Study the drawing (mm; zero at the part's minimum x, y, z) and answer. A direction names the side the tool comes from. Round coordinates to 2 decimals unless told otherwise and drop trailing zeros. Loops run counter-clockwise (first coordinate to the right, second up) from the corner with the lowest first, then second, coordinate; pieces in that order, holes last. Notation, with made-up numbers: (-11, 7.25) - (4, 7.25) arc R30 ccw to (4, 31.25) - close; hole circle Ø7 at (2, 0.25). An arc over 180 degrees is marked (long way). Use CSV: the item, a comma, the result in double quotes. Start each with the question number.
1. Find section B-B (y = 56). Give the vertices of the cut face in (x, z).
2. Given pin 1 Ø10 at (y, z) = (83.5, 53.5) entering from +X; pin 2 Ø7.5 at (x, y) = (62.5, 46.5) entering from -Z; pin 3 Ø6 at (x, y) = (28.5, 19.5) entering from +Z; pin 4 Ø3.5 at (x, y) = (39.5, 7.5) entering from +Z, each flat-ended and moving along its own axis, determine where each tip first touches the part or whether it passes through.
3. Find section C-C (x = 36.5). Give the vertices of the cut face in (y, z), and give its area (3 significant figures).
4. Find section A-A (x = 12). Give the vertices of the cut face in (y, z), and give its area (3 significant figures).
5. A tool of negligible diameter and unlimited length cuts with its end or side. For the marked faces 1, 2 and 3, from which of +Z, -Z, +X, -X, +Y, -Y can it reach the whole face along a straight path? Write none if from no direction.
6. Consider line 1 along X through (y, z) = (94.5, 6); line 2 along Z through (x, y) = (43, 102); line 3 along Y through (x, z) = (25, 56.5). Determine where each line is inside the solid, lowest interval first.
7. Determine the mould class of the marked faces 4, 5 and 6 for opening direction Y: +Y half, -Y half, draft (parallel to the pull), parting line (faces both ways), or undercut.
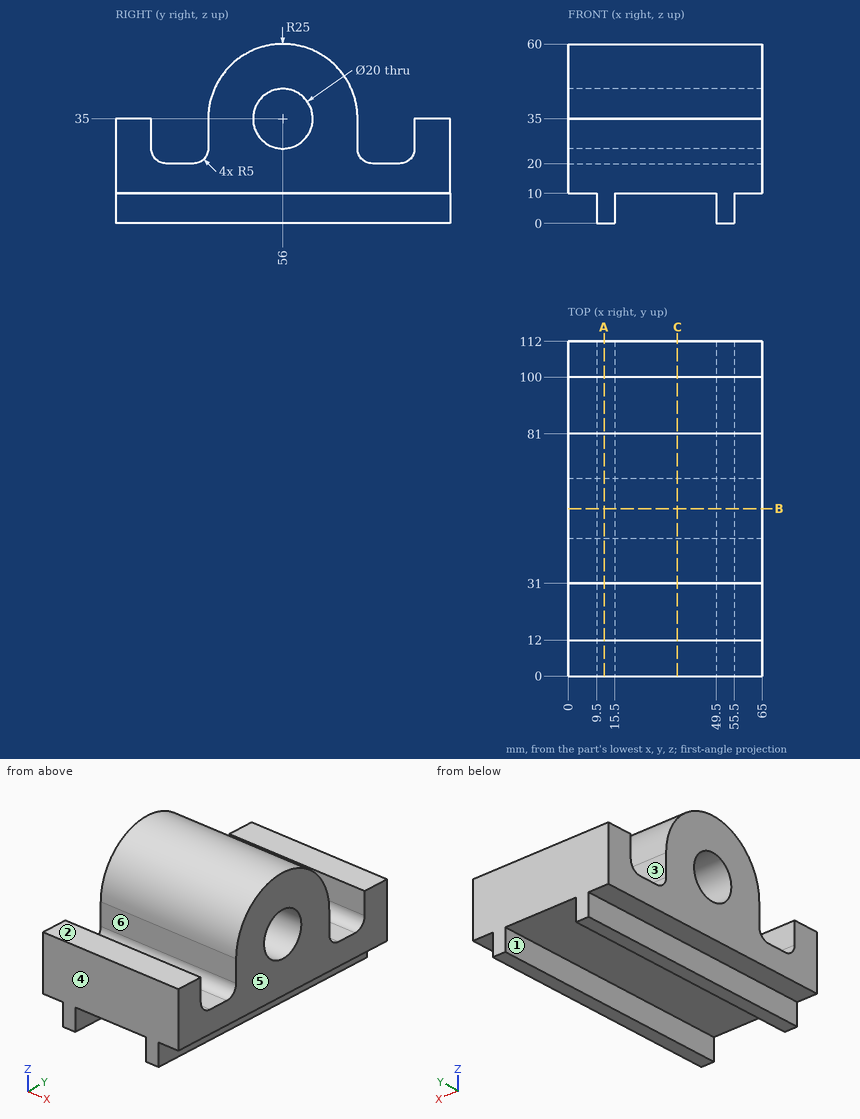
Filled sheet:
1,outline,"(0, 10) - (9.5, 10) - (9.5, 0) - (15.5, 0) - (15.5, 10) - (49.5, 10) - (49.5, 0) - (55.5, 0) - (55.5, 10) - (65, 10) - (65, 25) - (0, 25) - close; (0, 45) - (65, 45) - (65, 60) - (0, 60) - close"
2,pin 1,"passes through"
2,pin 2,"stops at z = 10"
2,pin 3,"stops at z = 20.03"
2,pin 4,"stops at z = 35"
3,outline,"(0, 10) - (112, 10) - (112, 35) - (100, 35) - (100, 25) arc R5 cw to (95, 20) - (86, 20) arc R5 cw to (81, 25) - (81, 35) arc R25 ccw to (31, 35) - (31, 25) arc R5 cw to (26, 20) - (17, 20) arc R5 cw to (12, 25) - (12, 35) - (0, 35) - close; hole circle Ø20 at (56, 35)"
3,area,"2,920 mm²"
4,outline,"(0, 0) - (112, 0) - (112, 35) - (100, 35) - (100, 25) arc R5 cw to (95, 20) - (86, 20) arc R5 cw to (81, 25) - (81, 35) arc R25 ccw to (31, 35) - (31, 25) arc R5 cw to (26, 20) - (17, 20) arc R5 cw to (12, 25) - (12, 35) - (0, 35) - close; hole circle Ø20 at (56, 35)"
4,area,"4,040 mm²"
5,face 1,"-Z, +Y, -Y"
5,face 2,"+Z, +X, -X, -Y"
5,face 3,"+Z, +X, -X"
6,line 1,"x = 9.5 to 15.5, 49.5 to 55.5"
6,line 2,"z = 10 to 35"
6,line 3,"y = 43.24 to 68.76"
7,face 4,"-Y half"
7,face 5,"draft"
7,face 6,"undercut"
